```python
from build123d import *

# Parameters (mm, degrees)
F0_R     = 25.4839572759
F1_DEPTH = 50.8
F2_R     = 10.16
F3_R     = 10.16
F4_T     = -2.54


# Not quite as in the source:
# - a shell that OpenCascade refuses in one call is made with other operations: the cavity is built on its own and cut out


with BuildPart() as f1:
    # F0 (on Top) → F1 (new body)
    with BuildSketch(Plane.XY):
        Circle(F0_R)
    extrude(amount=F1_DEPTH)

    # F2
    f2_edges = [f1.edges().sort_by_distance(p)[0] for p in [
        (-25.483957, 0, 0),
    ]]
    fillet(f2_edges, radius=F2_R)

    # F3
    f3_edges = [f1.edges().sort_by_distance(p)[0] for p in [
        (-25.483957, 0, 50.8),
    ]]
    fillet(f3_edges, radius=F3_R)

    # F4: a shell. OpenCascade refuses it in one call, so the cavity is built on its own and cut out:
    # the body offset inwards by the wall thickness, plus a prism from it out through each open face.
    f4_core = offset(f1.part, amount=F4_T, mode=Mode.PRIVATE)
    f4_exits = [f4_core.faces().sort_by_distance(p)[0] for p in [
        (0, 0, 48.26),
    ]]
    add(f4_core, mode=Mode.SUBTRACT)
    extrude(f4_exits, amount=-F4_T, mode=Mode.SUBTRACT)


solid = f1.part
```
CAD build for the part. Positions are in the model's coordinates, mm. A direction names the side the tool comes from. Coordinates: 2 decimals unless noted, no trailing zeros. Order: outer loops, then holes, each group sorted by start corner. A loop starts at its lowest first (then second) coordinate and runs counter-clockwise, first axis right, second up. Notation, with made-up numbers: (-23.75, -32.5) - (14.25, -32.5) arc R6 cw to (14.25, -28.5) - close; hole circle Ø6 at (70, 36.25). An arc over 180 degrees is marked (long way). Use a Markdown table: item, result. Add a question column.
(1) Which spindle directions (+Z, -Z, +X, -X, +Y, -Y) get a long thin tool onto all of the face, cutting with end or side? Do faces 4 (the face through (14.616, 4.603, 49.512)), 5 (the face through (21.884, 6.892, 25.187)). Say none if no direction does.
(2) Pull direction Y, two halves, no side cores. Call faces 1 (the face through (0, 0, 0)), 2 (the face through (0, 0, 2.54)), 3 (the face through (-5.52, -24.88, 25.19)): +Y half, -Y half, draft (parallel to the pull), parting line (faces both ways), or undercut.
(3) Saw through at A-A (y = 0). Give the cut face in (x, z).
(4) Saw through at C-C (z = 37). Give the cut face in (x, y), then the cut area to 3 significant figures.
(5) Flat gauge pins, fed straight in: pin 1 (2 mm diameter, centred on x = -14, z = 19.5, fed in from +Y); pin 2 (10 mm diameter, centred on x = 0.5, y = -16.5, fed in from +Z); pin 3 (1 mm diameter, centred on y = -19, z = 37, fed in from +X); pin 4 (1 mm diameter, centred on y = -1, z = 13, fed in from +X). Where does each tip first touch, or does it go through?
(6) Drill centre lines: line 1 along Y through (x, z) = (0, 19); line 2 along Z through (x, y) = (1.5, -8.5). Where is each one in solid material? Low to high. Write a range as [from, to].
Solved:
| question | item | result |
|---|---|---|
| 1 | face 4 | +Z |
| 1 | face 5 | none |
| 2 | face 1 | draft |
| 2 | face 2 | undercut |
| 2 | face 3 | parting line |
| 3 | outline | (-25.48, 10.16) arc R10.16 ccw to (-15.32, 0) - (15.32, 0) arc R10.16 ccw to (25.48, 10.16) - (25.48, 40.64) arc R10.16 ccw to (15.32, 50.8) - (15.32, 48.26) arc R7.62 cw to (22.94, 40.64) - (22.94, 10.16) arc R7.62 cw to (15.32, 2.54) - (-15.32, 2.54) arc R7.62 cw to (-22.94, 10.16) - (-22.94, 40.64) arc R7.62 cw to (-15.32, 48.26) - (-15.32, 50.8) arc R10.16 ccw to (-25.48, 40.64) - close |
| 4 | outline | circle Ø50.97 at (0, 0); hole circle Ø45.89 at (0, 0) |
| 4 | area | 386 mm² |
| 5 | pin 1 | stops at y = 21.92 |
| 5 | pin 2 | stops at z = 50.8 |
| 5 | pin 3 | stops at x = 17.53 |
| 5 | pin 4 | stops at x = 25.48 |
| 6 | line 1 | y = [-25.48, -22.94], [22.94, 25.48] |
| 6 | line 2 | z = [0, 2.54] |
